Job drawing, mm, ordinate dimensions from the low corner. One solid piece. Give positions to 0.01 mm unless a question says otherwise; leave off trailing zeros. Order: outer loops, then holes, each group sorted by start corner. A loop starts at its lowest first (then second) coordinate and runs counter-clockwise, first axis right, second up.
Item 1: Band-saw the part on A-A on y = 7.25. Give the cut face in (x, z), plus the area to 3 significant figures.
Item 2: Two-plate mould, pull along Z, no slides. Class the marked faces 1 and 2: released by +Z, released by -Z, zero draft, split by the parting line, or undercut.
Item 3: Flat gauge pins, fed straight in: P1, Ø0.8, axis at y = 6, z = 48.5, coming from the +X side; P2, Ø5.5, axis at x = 103, y = 8, coming from the -Z side; P3, Ø3, axis at y = 5, z = 49.5, coming from the -X side; P4, Ø3, axis at y = 8.5, z = 16, coming from the -X side. Where does each tip first touch, or does it go through?
Item 4: Band-saw the part on B-B on x = 66. Give the cut face in (y, z).
Item 5: Wall check: L1, parallel to Z at x = 100.7, y = 4.25; L2, parallel to X at y = 5.75, z = 9.3; L3, parallel to Z at x = 100, y = 6.25. Give the ranges that are in metal, low to high.
Item 6: Band-saw the part on D-D on x = 100.7. Give the cut face in (y, z), plus the area to 3 significant figures.
Item 7: Band-saw the part on C-C on z = 35.5. Give the cut face in (x, y).
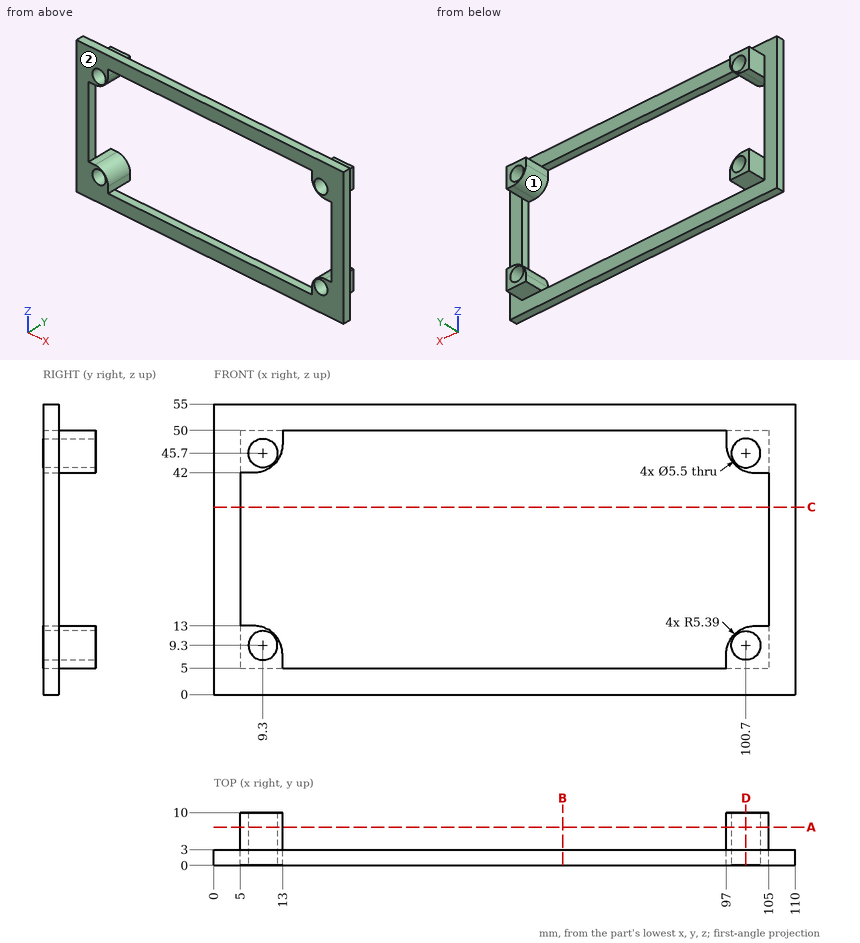
The answers:
1. outline: (5, 5) - (13, 5) - (13, 7.61) arc R5.39 ccw to (7.61, 13) - (5, 13) - close; (5, 42) - (7.61, 42) arc R5.39 ccw to (13, 47.39) - (13, 50) - (5, 50) - close; (97, 5) - (105, 5) - (105, 13) - (102.39, 13) arc R5.39 ccw to (97, 7.61) - close; (97, 47.39) arc R5.39 ccw to (102.39, 42) - (105, 42) - (105, 50) - (97, 50) - close; hole circle Ø5.5 at (9.3, 9.3); hole circle Ø5.5 at (9.3, 45.7); hole circle Ø5.5 at (100.7, 9.3); hole circle Ø5.5 at (100.7, 45.7)
1. area: 136 mm2
2. face 1: undercut
2. face 2: zero draft
3. P1: stops at x = 105
3. P2: stops at z = 5
3. P3: stops at x = 5
3. P4: passes through
4. outline: (0, 0) - (3, 0) - (3, 5) - (0, 5) - close; (0, 50) - (3, 50) - (3, 55) - (0, 55) - close
5. L1: z = 5 to 6.55, 12.05 to 12.73, 42.27 to 42.95, 48.45 to 50
5. L2: x = 5 to 6.55, 12.05 to 12.73, 97.27 to 97.95, 103.45 to 105
5. L3: z = 5 to 6.64, 11.96 to 12.44, 42.56 to 43.04, 48.36 to 50
6. outline: (0, 0) - (3, 0) - (3, 5) - (10, 5) - (10, 6.55) - (0, 6.55) - close; (0, 12.05) - (10, 12.05) - (10, 12.73) - (0, 12.73) - close; (0, 42.27) - (10, 42.27) - (10, 42.95) - (0, 42.95) - close; (0, 48.45) - (10, 48.45) - (10, 50) - (3, 50) - (3, 55) - (0, 55) - close
6. area: 74.6 mm2
7. outline: (0, 0) - (5, 0) - (5, 3) - (0, 3) - close; (105, 0) - (110, 0) - (110, 3) - (105, 3) - close
